Geometry: final body of the model. Coordinates: model frame, mm. Face numbers are marked on the shaded views. A direction names the side the tool comes from. Round coordinates to 2 decimals unless told otherwise and drop trailing zeros. Order: outer loops, then holes, each group sorted by start corner. A loop starts at its lowest first (then second) coordinate and runs counter-clockwise, first axis right, second up. Notation, with made-up numbers: M 89,-38 L 123,-38 A28 ccw 123,-10 Z; hole C -29.5,83.5 d4. An arc over 180 degrees is marked long. Put each result on its own line as item: value. Start each with the question number.
1) Section B-B, the plane x = -147. Return loops of the section in (y, z).
2) Access query for the marked faces 1, 2, 3, 4 and 5. Directions: +Z, -Z, +X, -X, +Y, -Y. A direction counts if a zero-diameter tool reaches every point of the face in a straight line with its end or side. Return the directions, or none.
3) Section D-D, the plane z = 4. Return loops of the section in (x, y), then the cut area to 3 significant figures.
4) Material intervals for probe 1 along X at (y, z) = (2.5, 49); probe 2 along X at (y, z) = (-1, 26); probe 3 along Z at (x, y) = (-131.25, -25), sorted ascending. Write a range as [from, to].
5) Section A-A, the plane y = 0. Return loops of the section in (x, z).
6) First-contact query: P1, Ø0.8, axis at x = -154, z = 28, coming from the +Y side; P2, Ø3, axis at x = -165, z = 31, coming from the -Y side; P3, Ø12.5, axis at y = -5.5, z = 35, coming from the -X side; P4, Ø10, axis at x = -147.5, y = 30, coming from the +Z side. Flat tips, straight axial feed; report the tip coordinate or a pass-through.
7) Draft query along X for the marked faces 6, 7 and 8. Return one class per face: pulls with the +X half, pulls with the -X half, needs draft (parallel to the pull), parting line crosses it, or undercut.
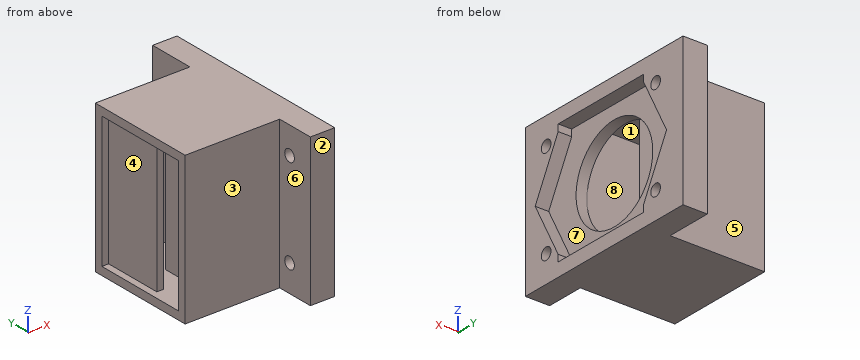
from build123d import *

# Parameters (mm, degrees)
SKETCH044_W     = 72
SKETCH044_H     = 55
PAD022_DEPTH    = 4
SKETCH046_R     = 17.5
POCKET015_DEPTH = 4.001
SKETCH047_W     = 72
SKETCH047_H     = 55
PAD023_DEPTH    = 5
SKETCH045_R     = 2.2
HOLE007_DEPTH   = 25
SKETCH048_W     = 41
SKETCH048_H     = 55
SKETCH048_W_2   = 35
SKETCH048_H_2   = 49
PAD024_DEPTH    = 35
SKETCH049_W     = 22
SKETCH049_H     = 2.5
PAD025_DEPTH    = 49


with BuildPart() as part:
    # Sketch044 → Pad022 (new body)
    with BuildSketch(Plane.YZ.offset(-130)):
        with Locations((1.5, 27.5)):
            Rectangle(SKETCH044_W, SKETCH044_H)
    extrude(amount=-PAD022_DEPTH)

    # Sketch046 (on Face5 of Hole007) → Pocket015 (cut, through all)
    with BuildSketch(Plane(origin=(-134, 0, 0), x_dir=(0, 1, 0), z_dir=(-1, 0, 0))):
        with Locations((0, -27.5)):
            Circle(SKETCH046_R)
    extrude(amount=-POCKET015_DEPTH, mode=Mode.SUBTRACT)

    # Sketch047 (on Face4 of Pocket015) → Pad023 (join)
    with BuildSketch(Plane.YZ.offset(-130)):
        with Locations((1.5, 27.5)):
            Rectangle(SKETCH047_W, SKETCH047_H)
        Polygon((-30, 27.5), (-19.5, 7.5), (-19.5, 5), (19.5, 5), (19.5, 7.5), (30, 27.5), (19.5, 47.5), (19.5, 50), (-19.5, 50), (-19.5, 47.5), align=None, mode=Mode.SUBTRACT)
    extrude(amount=PAD023_DEPTH)

    # Sketch045 (on Face6 of Pad022) → Hole007 (cut)
    with BuildSketch(Plane(origin=(-134, 0, 0), x_dir=(0, 1, 0), z_dir=(-1, 0, 0))):
        with Locations((-25, -10)):
            Circle(SKETCH045_R)
        with Locations((-25, -45)):
            Circle(SKETCH045_R)
        with Locations((25, -45)):
            Circle(SKETCH045_R)
        with Locations((25, -10)):
            Circle(SKETCH045_R)
    extrude(amount=-HOLE007_DEPTH, mode=Mode.SUBTRACT)

    # Sketch048 (on Face5 of Hole007) → Pad024 (join)
    with BuildSketch(Plane(origin=(-134, 0, 0), x_dir=(0, 1, 0), z_dir=(-1, 0, 0))):
        with Locations((0, -27.5)):
            Rectangle(SKETCH048_W, SKETCH048_H)
        with Locations((0, -27.5)):
            Rectangle(SKETCH048_W_2, SKETCH048_H_2, mode=Mode.SUBTRACT)
    extrude(amount=PAD024_DEPTH)

    # Sketch049 (on Face31 of Pad024) → Pad025 (join)
    with BuildSketch(Plane(origin=(0, 0, 3), x_dir=(0, -1, 0), z_dir=(0, 0, 1))):
        with Locations((-6.5, -144.25)):
            Rectangle(SKETCH049_W, SKETCH049_H)
        with Locations((6.5, -154.75)):
            Rectangle(SKETCH049_W, SKETCH049_H)
        with Locations((-6.5, -165.25)):
            Rectangle(SKETCH049_W, SKETCH049_H)
    extrude(amount=PAD025_DEPTH)


solid = part.part
Result sheet:
1. outline: M -20.5,0 L 20.5,0 L 20.5,55 L -20.5,55 Z; hole M -17.5,3 L 17.5,3 L 17.5,52 L -17.5,52 Z
2. face 1: none
2. face 2: +Z, -Z, +X, -X, -Y
2. face 3: +Z, -Z, -X, -Y
2. face 4: -X
2. face 5: +Z, -Z, -X, +Y
3. outline: M -169,-20.5 L -134,-20.5 L -134,-34.5 L -125,-34.5 L -125,37.5 L -134,37.5 L -134,20.5 L -169,20.5 L -169,17.5 L -166.5,17.5 L -166.5,-4.5 L -164,-4.5 L -164,17.5 L -145.5,17.5 L -145.5,-4.5 L -143,-4.5 L -143,17.5 L -134,17.5 L -134,-17.5 L -153.5,-17.5 L -153.5,4.5 L -156,4.5 L -156,-17.5 L -169,-17.5 Z
3. area: 1,020 mm2
4. probe 1: x = [-166.5, -164], [-156, -153.5], [-145.5, -143], [-134, -130]
4. probe 2: x = [-166.5, -164], [-156, -153.5], [-145.5, -143]
4. probe 3: z = [0, 7.8], [12.2, 42.8], [47.2, 55]
5. outline: M -169,0 L -125,0 L -125,5 L -130,5 L -130,10 L -134,10 L -134,3 L -143,3 L -143,52 L -134,52 L -134,45 L -130,45 L -130,50 L -125,50 L -125,55 L -169,55 L -169,52 L -166.5,52 L -166.5,3 L -169,3 Z; hole M -164,3 L -156,3 L -156,52 L -164,52 Z; hole M -153.5,3 L -145.5,3 L -145.5,52 L -153.5,52 Z
6. P1: stops at y = 20.5
6. P2: stops at y = -20.5
6. P3: stops at x = -166.5
6. P4: passes through
7. face 6: pulls with the -X half
7. face 7: pulls with the +X half
7. face 8: undercut
